```python
from build123d import *

# Parameters (mm, degrees)
F1_DEPTH  = 7.5
F5_DEPTH  = 10
F6_DEPTH  = 70
F7_W      = 15
F7_H      = 10
F8_DEPTH  = 70
F9_DEPTH  = 70
F10_W     = 10
F10_H     = 85
F11_DEPTH = 70


with BuildPart() as f1:
    # F0 (on Front) → F1 (new body, symmetric)
    with BuildSketch(Plane.XZ):
        with BuildLine():
            ThreePointArc((-27.5296741368, 14.9347687151), (-34.9790626376, -16.4884870212), (-27.5296741368, -47.9117427575))
            Line((-27.5296741368, -47.9117427575), (-12.5296741368, -47.9117427575))
            ThreePointArc((-12.5296741368, -47.9117427575), (-5.0802856361, -16.4884870212), (-12.5296741368, 14.9347687151))
            Line((-12.5296741368, 14.9347687151), (-27.5296741368, 14.9347687151))
        make_face()
    extrude(amount=F1_DEPTH, both=True)


with BuildPart() as f2_1:
    # F2: copy of F1
    add(f1.part.moved(Location((70, 0, 0))))


with BuildPart() as f3_1:
    # F3: copy of F1
    add(f1.part.moved(Location((0, 70, 0))))


with BuildPart() as f4_1:
    # F4: copy of F2_1
    add(f2_1.part.moved(Location((0, 70, 0))))


with BuildPart() as f1_1:
    add(f1.part)

    # F5 (add): a face of the model
    f5_faces = [f1_1.faces().sort_by_distance(p)[0] for p in [
        (-20.0296741368, 0, 14.9347687151),
    ]]
    extrude(f5_faces, amount=F5_DEPTH)

    # F6 (add): a face of the model
    f6_faces = [f1_1.faces().sort_by_distance(p)[0] for p in [
        (-12.5296741368, 0, 19.9347687151),
    ]]

    add(f2_1.part)  # F6 merges F2_1
    extrude(f6_faces, amount=F6_DEPTH)

    add(f4_1.part)  # F8 merges F4_1
    # F7 (on face) → F8 (join)
    with BuildSketch(Plane(origin=(0, 7.5, 0), x_dir=(-1, 0, 0), z_dir=(0, 1, 0))):
        with Locations((-49.9703258632, 19.9347687151)):
            Rectangle(F7_W, F7_H)
    extrude(amount=F8_DEPTH)

    # F9 (add): a face of the model
    f9_faces = [f1_1.faces().sort_by_distance(p)[0] for p in [
        (42.4703258632, 42.5, 19.9347687151),
    ]]

    add(f3_1.part)  # F9 merges F3_1
    extrude(f9_faces, amount=F9_DEPTH)

    # F10 (on face) → F11 (join)
    with BuildSketch(Plane.XY.offset(24.9347687151)):
        with Locations((-22.5296741368, 35)):
            Rectangle(F10_W, F10_H)
    extrude(amount=F11_DEPTH)


solid = f1_1.part
```
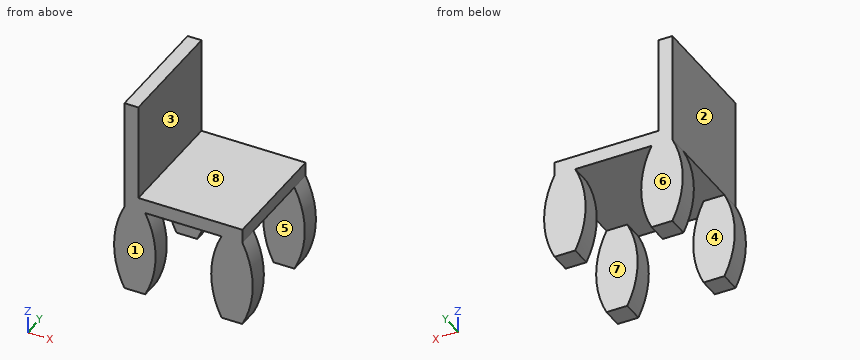
Verification items for the finished model (mm, model axes). Face numbers are marked on the shaded views. A direction names the side the tool comes from. Round coordinates to 2 decimals unless told otherwise and drop trailing zeros. Order: outer loops, then holes, each group sorted by start corner. A loop starts at its lowest first (then second) coordinate and runs counter-clockwise, first axis right, second up. Notation, with made-up numbers: (18.25, 13) -> (68.25, 13) arc R18 ccw to (68.25, 37) -> close; hole circle Ø3 at (70, -5). An arc over 180 degrees is marked (long way). Put each result on its own line as item: value. Start each with the question number.
(1) Draft check along Y on the marked faces 5, 6, 7 and 8. Enter one of: +Y half, -Y half, draft (parallel to the pull), parting line (faces both ways), or undercut.
(2) Section check D-D (z = -24). Enter the section's corners in (x, y).
(3) Tool access check on the marked faces 1, 2, 3 and 4. Record the directions out of +Z, -Z, +X, -X, +Y, -Y that give a thin tool (end or side, any length) a straight path to the whole face; none if there is none.
(4) Depth check by flat-ended pin: pin 1 Ø4 at (y, z) = (68, 54.5) entering from +X; pin 2 Ø1 at (y, z) = (29, 72) entering from -X; pin 3 Ø22.5 at (x, y) = (35, 20) entering from +Z; pin 4 Ø8 at (x, z) = (-2, 28.5) entering from +Y. Enter the tip coordinate at first touch or a pass-through.
(5) Material ranges on line 1 along Y through (x, z) = (-8, -23.5); line 2 along Z through (x, y) = (4, 66.5); line 3 along X through (y, z) = (53, 34), recorded low to high.
(6) Section check A-A (z = 7.5). Enter the section's corners in (x, y).
(7) Section check B-B (y = 4.5). Enter the section's corners in (x, z).
(8) Section check C-C (x = 51.5). Enter the section's corners in (y, z), then the cut area to 3 significant figures.
Completed:
1. face 5: undercut
1. face 6: +Y half
1. face 7: undercut
1. face 8: draft
2. outline: (-34.57, -7.5) -> (-5.48, -7.5) -> (-5.48, 7.5) -> (-34.57, 7.5) -> close; (-34.57, 62.5) -> (-5.48, 62.5) -> (-5.48, 77.5) -> (-34.57, 77.5) -> close; (35.43, -7.5) -> (64.52, -7.5) -> (64.52, 7.5) -> (35.43, 7.5) -> close; (35.43, 62.5) -> (64.52, 62.5) -> (64.52, 77.5) -> (35.43, 77.5) -> close
3. face 1: +Z, -Z, +X, -X, -Y
3. face 2: +Z, -X, +Y, -Y
3. face 3: +Z, +X, +Y, -Y
3. face 4: -Z, +X, -X
4. pin 1: stops at x = -17.53
4. pin 2: stops at x = -27.53
4. pin 3: stops at z = 24.93
4. pin 4: stops at y = 77.5
5. line 1: y = -7.5 to 7.5, 62.5 to 77.5
5. line 2: z = 14.93 to 24.93
5. line 3: x = -27.53 to -17.53
6. outline: (-30.74, -7.5) -> (-9.32, -7.5) -> (-9.32, 7.5) -> (-30.74, 7.5) -> close; (-30.74, 62.5) -> (-9.32, 62.5) -> (-9.32, 77.5) -> (-30.74, 77.5) -> close; (39.26, -7.5) -> (60.68, -7.5) -> (60.68, 7.5) -> (39.26, 7.5) -> close; (39.26, 62.5) -> (60.68, 62.5) -> (60.68, 77.5) -> (39.26, 77.5) -> close
7. outline: (-27.53, -47.91) -> (-12.53, -47.91) arc R70 ccw to (-12.53, 14.93) -> (42.47, 14.93) arc R70 ccw to (42.47, -47.91) -> (57.47, -47.91) arc R70 ccw to (57.47, 14.93) -> (57.47, 24.93) -> (-17.53, 24.93) -> (-17.53, 94.93) -> (-27.53, 94.93) -> (-27.53, 14.93) arc R70 ccw to start
8. outline: (-7.5, -47.91) -> (7.5, -47.91) -> (7.5, 14.93) -> (62.5, 14.93) -> (62.5, -47.91) -> (77.5, -47.91) -> (77.5, 24.93) -> (-7.5, 24.93) -> close
8. area: 2,740 mm2
